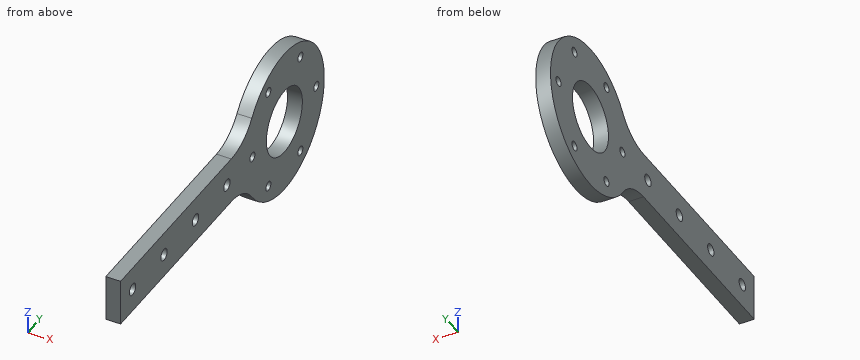
from build123d import *

# Parameters (mm, degrees)
BOSS_EXTRUDE1_DEPTH = 6.35
FILLET1_R           = 20
SKETCH2_R           = 14.3
SKETCH2_R_2         = 2
CUT_EXTRUDE1_DEPTH  = 7.35
SKETCH3_R           = 2.525
CUT_EXTRUDE2_DEPTH  = 7.35


with BuildPart() as part:
    # Sketch1 → Boss-Extrude1 (new body)
    with BuildSketch(Plane(origin=(0, 0, 0), x_dir=(0, 0, -1), z_dir=(1, 0, 0))):
        with BuildLine():
            Line((-10, -30.134075396), (-10, -130.134075396))
            Line((-10, -130.134075396), (10, -130.134075396))
            Line((10, -130.134075396), (10, -30.134075396))
            ThreePointArc((10, -30.134075396), (0, 31.75), (-10, -30.134075396))
        make_face()
    extrude(amount=BOSS_EXTRUDE1_DEPTH)

    # Fillet1
    fillet1_edges = [part.edges().sort_by_distance(p)[0] for p in [
        (3.175, -30.134075396, -10),
        (3.175, -30.134075396, 10),
    ]]
    fillet(fillet1_edges, radius=FILLET1_R)

    # Sketch2 → Cut-Extrude1 (cut, through all)
    with BuildSketch(Plane(origin=(6.35, 0, 0), x_dir=(0, 0, -1), z_dir=(1, 0, 0))):
        Circle(SKETCH2_R)
        with Locations((0, 25.4)):
            Circle(SKETCH2_R_2)
        with Locations((21.997045256, 12.7)):
            Circle(SKETCH2_R_2)
        with Locations((21.997045256, -12.7)):
            Circle(SKETCH2_R_2)
        with Locations((0, -25.4)):
            Circle(SKETCH2_R_2)
        with Locations((-21.997045256, -12.7)):
            Circle(SKETCH2_R_2)
        with Locations((-21.997045256, 12.7)):
            Circle(SKETCH2_R_2)
    extrude(amount=-CUT_EXTRUDE1_DEPTH, mode=Mode.SUBTRACT)

    # Sketch3 → Cut-Extrude2 (cut, through all)
    with BuildSketch(Plane(origin=(6.35, 0, 0), x_dir=(0, 0, -1), z_dir=(1, 0, 0))):
        with Locations((0, -120.63662428)):
            Circle(SKETCH3_R)
        with Locations((0, -95.63662428)):
            Circle(SKETCH3_R)
        with Locations((0, -70.63662428)):
            Circle(SKETCH3_R)
        with Locations((0, -45.63662428)):
            Circle(SKETCH3_R)
    extrude(amount=-CUT_EXTRUDE2_DEPTH, mode=Mode.SUBTRACT)


solid = part.part
Source: CAD feature listing. Evaluate the final solid. Frame: model axes, mm. Round coordinates to 2 decimals unless told otherwise and drop trailing zeros. Loops run counter-clockwise (first coordinate to the right, second up) from the corner with the lowest first, then second, coordinate; pieces in that order, holes last. Notation, with made-up numbers: M 82,-13 L 93,-13 A22 cw 93,22 Z; hole C 30.5,27.5 d8. An arc over 180 degrees is marked long. Return JSON: item names as keys, results as strings. Group by question number.
1. Section query B-B on z = 0. State how many separate pieces and enclosed holes the cut face has, and give its area (3 significant figures).
2. Section query A-A on y = 0. Output: boundary loops of the cut face in (x, z).
3. Pin query (flat end, axial travel): pin 1 (2.5 mm diameter, centred on y = 25.4, z = 0, fed in from +X); pin 2 (6 mm diameter, centred on y = -95.64, z = 0, fed in from +X); pin 3 (1.5 mm diameter, centred on x = 1.5, z = 21, fed in from +Y); pin 4 (1 mm diameter, centred on x = 4.5, y = -2.5, fed in from +Z). Return the tip coordinate at first contact, or that it passes through.
4. Material intervals for line 1 along Y through (x, z) = (4.25, 21); line 2 along Y through (x, z) = (6.25, 21.5); line 3 along Y through (x, z) = (2.5, -6), sorted ascending. Write a range as from..to.
5. Section query C-C on y = 25.4. Output: boundary loops of the cut face in (x, z), and give its area (3 significant figures).
Checks:
{
 "1": {"separate pieces": "8", "enclosed holes": "0", "area": "667 mm²"},
 "2": {"outline": "M 0,-31.75 L 6.35,-31.75 L 6.35,-14.3 L 0,-14.3 Z; M 0,14.3 L 6.35,14.3 L 6.35,31.75 L 0,31.75 Z"},
 "3": {"pin 1": "passes through", "pin 2": "stops at x = 6.35", "pin 3": "stops at y = 24.45", "pin 4": "stops at z = 31.69"},
 "4": {"line 1": "y = -23.81..-14.43, -10.97..10.97, 14.43..23.81", "line 2": "y = -23.36..-14.64, -10.76..10.76, 14.64..23.36", "line 3": "y = -130.13..-12.98, 12.98..31.18"},
 "5": {"outline": "M 0,-19.05 L 6.35,-19.05 L 6.35,-2 L 0,-2 Z; M 0,2 L 6.35,2 L 6.35,19.05 L 0,19.05 Z", "area": "217 mm²"}
}
